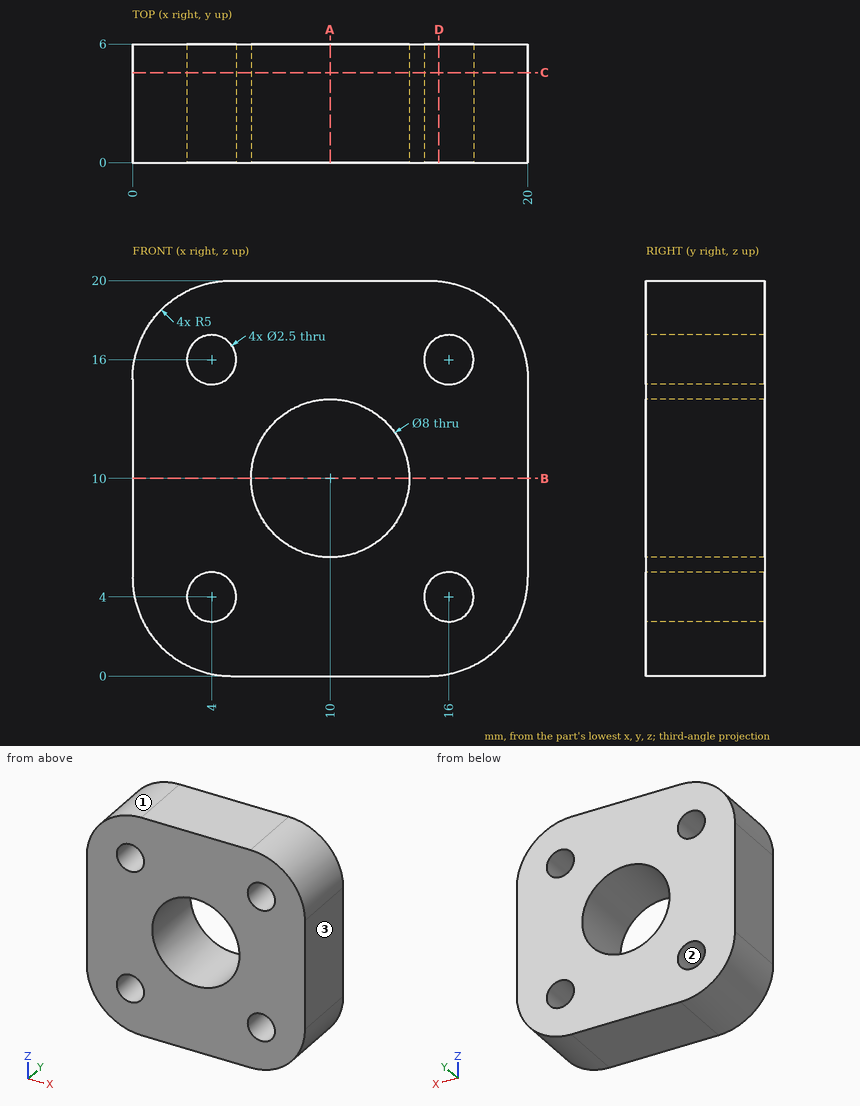
For this review, use the dimensioned drawing (mm, ordinates from the lowest corner) and the shaded views. Round coordinates to 2 decimals unless told otherwise and drop trailing zeros. Write each loop counter-clockwise with the first axis right and the second up, starting at its lowest first coordinate (ties: lowest second). Pieces come first, ordered by that corner, then holes. Notation, with made-up numbers: (-4.5, 73.5) -> (13.5, 73.5) arc R8 cw to (13.5, 88.5) -> close; hole circle Ø5 at (67.25, 48). An arc over 180 degrees is marked (long way). Use CSV: the item, a comma, the result in double quotes.
(1) Draft analysis for pull direction X (two halves, no side actions). For the marked faces 1, 2 and 3, state which applies: +X half, -X half, draft (parallel to the pull), parting line (faces both ways), or undercut.
Computed values:
face 1,"-X half"
face 2,"undercut"
face 3,"+X half"
(2) Consider section A-A, the plane x = 10. Give the boundary of the cut face in (y, z).
Computed values:
outline,"(0, 0) -> (6, 0) -> (6, 6) -> (0, 6) -> close; (0, 14) -> (6, 14) -> (6, 20) -> (0, 20) -> close"
(3) To check wall thickness, follow L1, parallel to Z at x = 16, y = 4.8; L2, parallel to Z at x = 15.5, y = 3.9. State the ranges of each line that lie inside material, in increasing order. Write a range as [from, to].
Computed values:
L1,"[0.1, 2.75], [5.25, 14.75], [17.25, 19.9]"
L2,"[0.03, 2.85], [5.15, 14.85], [17.15, 19.97]"
(4) Consider section C-C, the plane y = 4.55. Give the boundary of the cut face in (x, z), plus the area to 3 significant figures.
Computed values:
outline,"(0, 5) arc R5 ccw to (5, 0) -> (15, 0) arc R5 ccw to (20, 5) -> (20, 15) arc R5 ccw to (15, 20) -> (5, 20) arc R5 ccw to (0, 15) -> close; hole circle Ø2.5 at (4, 4); hole circle Ø2.5 at (4, 16); hole circle Ø8 at (10, 10); hole circle Ø2.5 at (16, 4); hole circle Ø2.5 at (16, 16)"
area,"309 mm²"
(5) Consider section B-B, the plane z = 10. Give the boundary of the cut face in (x, y), plus the area to 3 significant figures.
Computed values:
outline,"(0, 0) -> (6, 0) -> (6, 6) -> (0, 6) -> close; (14, 0) -> (20, 0) -> (20, 6) -> (14, 6) -> close"
area,"72.0 mm²"
(6) Consider section D-D, the plane x = 15.5. Give the boundary of the cut face in (y, z), plus the area to 3 significant figures.
Computed values:
outline,"(0, 0.03) -> (6, 0.03) -> (6, 2.85) -> (0, 2.85) -> close; (0, 5.15) -> (6, 5.15) -> (6, 14.85) -> (0, 14.85) -> close; (0, 17.15) -> (6, 17.15) -> (6, 19.97) -> (0, 19.97) -> close"
area,"92.2 mm²"
